```python
from build123d import *

# Parameters (mm, degrees)
F1_DEPTH = 101.6
F3_DEPTH = 76.2
F4_R     = 6.35


with BuildPart() as f1:
    # F0 (on Front) → F1 (new body)
    with BuildSketch(Plane.XZ):
        Polygon((-21.789443, 50.194677), (-97.989443, 50.194677), (-72.589443, -51.405323), (79.810557, -51.405323), (105.210557, 50.194677), (29.010557, 50.194677), (18.30329, 33.187184), (18.30329, 20.498006), (12.626553, 12.483789), (12.626553, -6.216054), (0.295312, -25.542488), (-0.553554, -4.574321), (-11.90842, 10.283374), (-12.26442, 20.09797), (-19.969508, 30.179977), align=None)
    extrude(amount=F1_DEPTH)

    # F2 (on Front) → F3 (cut)
    with BuildSketch(Plane.XZ):
        with BuildLine():
            Line((-49.430657, 37.494677), (-81.723583, 37.494677))
            Line((-81.723583, 37.494677), (-62.673583, -38.705323))
            Line((-62.673583, -38.705323), (-11.882212, -38.705323))
            Line((-11.882212, -38.705323), (0, -24.789929))
            Line((0, -24.789929), (6.961702, -38.705323))
            Line((6.961702, -38.705323), (69.894697, -38.705323))
            Line((69.894697, -38.705323), (88.944697, 37.494677))
            Line((88.944697, 37.494677), (36.022353, 37.494677))
            ThreePointArc((36.022353, 37.494677), (27.04006, 36.48556), (18.505591, 33.508521))
            Line((18.505591, 33.508521), (-19.994486, 30.454669))
            ThreePointArc((-19.994486, 30.454669), (-34.271665, 35.818222), (-49.430657, 37.494677))
        make_face()
    extrude(amount=F3_DEPTH, mode=Mode.SUBTRACT)

    # F4
    f4_edges = [f1.edges().sort_by_distance(p)[0] for p in [
        (-11.882212, -38.1, -38.705323),
        (6.961702, -38.1, -38.705323),
        (-62.673583, -38.1, -38.705323),
        (69.894697, -38.1, -38.705323),
        (88.944697, -38.1, 37.494677),
        (-81.723583, -38.1, 37.494677),
    ]]
    fillet(f4_edges, radius=F4_R)


solid = f1.part
```
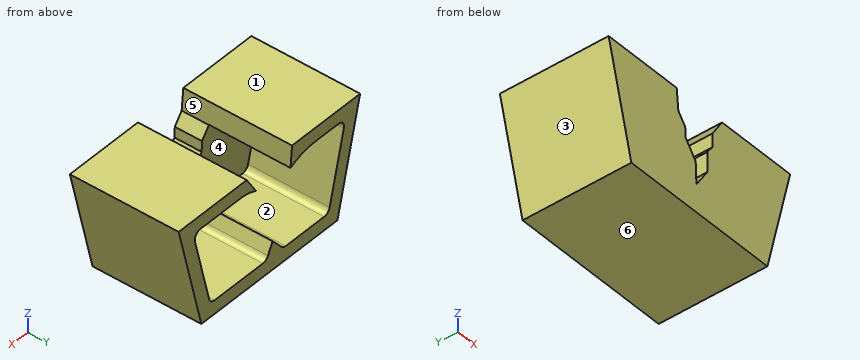
The listing builds one solid part. Answer for the finished solid, in the listing's coordinates (mm). Face numbers are marked on the shaded views. A direction names the side the tool comes from. Coordinates: 2 decimals unless noted, no trailing zeros. Write each loop counter-clockwise with the first axis right and the second up, starting at its lowest first coordinate (ties: lowest second). Pieces come first, ordered by that corner, then holes. Notation, with made-up numbers: (14, 6) - (41, 6) arc R27 ccw to (41, 23) - close; hole circle Ø2 at (13, 67.5). An arc over 180 degrees is marked (long way). Return JSON: item names as keys, results as strings. Group by question number.
1. Determine the mould class of the marked faces 1, 2 and 3 for opening direction Z: released by +Z, released by -Z, zero draft, split by the parting line, or undercut.
2. Straight lines are drawn through the part: L1, parallel to X at y = -30, z = -32.5; L2, parallel to Z at x = 53, y = -72; L3, parallel to X at y = -21.5, z = -29.5. For each, find the intervals that lie inside material, in ascending order.
3. Given pin 1 (1 mm diameter, centred on x = -52.5, z = 10.5, fed in from +Y); pin 2 (3 mm diameter, centred on y = -67.5, z = -6.5, fed in from -X); pin 3 (6 mm diameter, centred on y = -35.5, z = 23.5, fed in from +X), each flat-ended and moving along its own axis, determine where each tip first touches the part or whether it passes through.
4. A cutting plane is placed at B-B, the plane y = -21. Determine the outline of the cut face in (x, z), plus the area to 3 significant figures.
5. Which of the six approach directions +Z, -Z, +X, -X, +Y, -Y give full straight-line access (tool end or side, diameter ignored) to the marked faces 4, 5 and 6?
6. A cutting plane is placed at C-C, the plane x = -52. Determine the outline of the cut face in (y, z).
7. A cutting plane is placed at D-D, the plane y = -91.5. Determine the outline of the cut face in (x, z), plus the area to 3 significant figures.
8. A cutting plane is placed at A-A, the plane z = -22.5. Determine the outline of the cut face in (x, y).
Ans:
{
 "1": {"face 1": "released by +Z", "face 2": "undercut", "face 3": "released by -Z"},
 "2": {"L1": "-77.32 to -64.22, -6.58 to 3.86, 71.45 to 84.54", "L2": "-51.41 to -38.71, 37.49 to 50.19", "L3": "-78.07 to -64.97, -4.02 to 2.36, 72.2 to 85.29"},
 "3": {"pin 1": "y = -76.2", "pin 2": "x = -84.19", "pin 3": "x = 99.29"},
 "4": {"outline": "(-97.99, 50.19) - (-72.59, -51.41) - (79.81, -51.41) - (105.21, 50.19) - (29.01, 50.19) - (18.51, 33.51) arc R40.48 cw to (36.02, 37.49) - (80.81, 37.49) arc R6.35 cw to (86.97, 29.6) - (71.1, -33.9) arc R6.35 cw to (64.94, -38.71) - (10.89, -38.71) arc R6.35 cw to (5.21, -35.2) - (0.34, -25.47) - (0.3, -25.54) - (0.29, -25.37) - (0, -24.79) - (-9.98, -36.48) arc R6.35 cw to (-14.81, -38.71) - (-57.72, -38.71) arc R6.35 cw to (-63.88, -33.9) - (-79.75, 29.6) arc R6.35 cw to (-73.59, 37.49) - (-49.43, 37.49) arc R61.36 cw to (-19.99, 30.45) - (-21.79, 50.19) - close", "area": "6,180 mm²"},
 "5": {"face 4": "+Y", "face 5": "+Z, +Y, -Y", "face 6": "-Z, +X, -X, +Y, -Y"},
 "6": {"outline": "(-101.6, -51.41) - (0, -51.41) - (0, -38.71) - (-76.2, -38.71) - (-76.2, 37.49) - (0, 37.49) - (0, 50.19) - (-101.6, 50.19) - close"},
 "7": {"outline": "(-97.99, 50.19) - (-72.59, -51.41) - (79.81, -51.41) - (105.21, 50.19) - (29.01, 50.19) - (18.3, 33.19) - (18.3, 20.5) - (12.63, 12.48) - (12.63, -6.22) - (0.3, -25.54) - (-0.55, -4.57) - (-11.91, 10.28) - (-12.26, 20.1) - (-19.97, 30.18) - (-21.79, 50.19) - close", "area": "16,200 mm²"},
 "8": {"outline": "(-79.82, -101.6) - (0.17, -101.6) - (0.17, -76.2) - (-66.72, -76.2) - (-66.72, 0) - (-79.82, 0) - close; (2.24, -101.6) - (87.04, -101.6) - (87.04, 0) - (73.95, 0) - (73.95, -76.2) - (2.24, -76.2) - close"}
}
